Part model, mm, in its own coordinate system. A direction names the side the tool comes from. Round coordinates to 2 decimals unless told otherwise and drop trailing zeros. Write each loop counter-clockwise with the first axis right and the second up, starting at its lowest first coordinate (ties: lowest second). Pieces come first, ordered by that corner, then holes.
```python
from build123d import *

# Parameters (mm, degrees)
F1_DEPTH = 63.5
F0_W     = 21.3821388448
F0_H     = 19.05
F2_DEPTH = 25.4
F3_DEPTH = 7.9375


with BuildPart() as f1:
    # F0 (on Front) → F1 (new body, symmetric)
    with BuildSketch(Plane.XZ):
        Polygon((-41.275, 9.525), (-41.275, -9.525), (41.275, -9.525), (41.275, 9.525), (22.225, 9.525), align=None)
    extrude(amount=F1_DEPTH, both=True)

    # F0 (on Front) → F2 (join, symmetric)
    with BuildSketch(Plane.XZ):
        with BuildLine():
            Line((22.225, 9.525), (41.275, 9.525))
            Line((41.275, 9.525), (41.275, 27.0002))
            ThreePointArc((41.275, 27.0002), (45.9246798487, 38.2255201513), (57.15, 42.8752))
            Line((57.15, 42.8752), (64.3428611552, 42.8752))
            Line((64.3428611552, 42.8752), (64.3428611552, 61.9252))
            Line((64.3428611552, 61.9252), (57.15, 61.9252))
            ThreePointArc((57.15, 61.9252), (32.4542956671, 51.6959043329), (22.225, 27.0002))
            Line((22.225, 27.0002), (22.225, 9.525))
        make_face()
        with Locations((75.0339305776, 52.4002)):
            Rectangle(F0_W, F0_H)
    extrude(amount=F2_DEPTH, both=True)

    # F0 (on Front) → F3 (join, symmetric)
    with BuildSketch(Plane.XZ):
        with BuildLine():
            add(Edge.make_bspline(
                [(-41.275, 9.525), (-41.1300323904, 24.9551124871), (18.149998039, 62.0910935104), (57.15, 61.9252)],
                knots=[0, 0, 0, 0, 111.5045361635, 111.5045361635, 111.5045361635, 111.5045361635], degree=3))
            Line((-41.275, 9.525), (22.225, 9.525))
            Line((22.225, 9.525), (22.225, 27.0002))
            ThreePointArc((22.225, 27.0002), (32.4542956671, 51.6959043329), (57.15, 61.9252))
        make_face()
    extrude(amount=F3_DEPTH, both=True)

    # F0 (on Front) → F4 (revolve)
    with BuildSketch(Plane.XZ):
        Polygon((85.725, 66.675), (85.725, 61.9252), (85.725, 42.8752), (85.725, 38.1), (115.1428611552, 38.1), (115.1428611552, 66.675), align=None)
    revolve(axis=Axis((85.725, 0, 52.3875), (0, 0, 1)))


solid = f1.part
```
Q1. Which spindle directions (+Z, -Z, +X, -X, +Y, -Y) get a long thin tool onto all of the face, cutting with end or side? Do faces 1 (the flat face through (41, 25.4, 36)), 2 (the flat face through (61, -20, 42.875)), 3 (the flat face through (41.275, -1, 4)), 4 (the flat face through (61, -20, 61.925)). Say none if no direction does.
Values follow:
face 1: +Z, -X, +Y
face 2: -Z, -Y
face 3: -Z, +X, +Y, -Y
face 4: +Z, -X, -Y
Q2. Cut at A-A on z = 6. Write the cut outline in (x, y) (3 decimals), plus the area to 3 significant figures.
Values follow:
outline: (-41.275, -63.5) - (41.275, -63.5) - (41.275, 63.5) - (-41.275, 63.5) - close
area: 10,500 mm2
Q3. Drop flat-ended pins along their axis: pin 1 (8 mm diameter, centred on x = 58, y = 28, fed in from -Z); pin 2 (4 mm diameter, centred on x = -13, y = -43.5, fed in from +Z) (3 decimals); pin 3 (4 mm diameter, centred on x = 67, y = -12, fed in from -Z). Give the stop position or say it passes through.
Values follow:
pin 1: stops at z = 42.72
pin 2: stops at z = 9.525
pin 3: stops at z = 38.1
Q4. Wall check: L1, parallel to Z at x = 86.5, y = -19 (3 decimals); L2, parallel to Y at x = 44, z = 37; L3, parallel to X at y = 19, z = 6 (3 decimals). Give the ranges that are in metal, low to high.
Values follow:
L1: z = 38.1 to 66.675
L2: y = -25.4 to 25.4
L3: x = -41.275 to 41.275
Q5. Cut at B-B on y = 49. Write the cut outline in (x, z) (3 decimals).
Values follow:
outline: (-41.275, -9.525) - (41.275, -9.525) - (41.275, 9.525) - (-41.275, 9.525) - close
Q6. Mould opens along X. For faces 5 (the cylindrical face through (45.8, -0.4, 38.1)), 6 (the flat face through (22.225, 17, 18)), 7 (the flat face through (86, 0, 38.1)), 8 (the flat face through (61, 20, 42.875)) say: +X half, -X half, draft (parallel to the pull), parting line (faces both ways), or undercut.
Values follow:
face 5: undercut
face 6: -X half
face 7: draft
face 8: undercut
